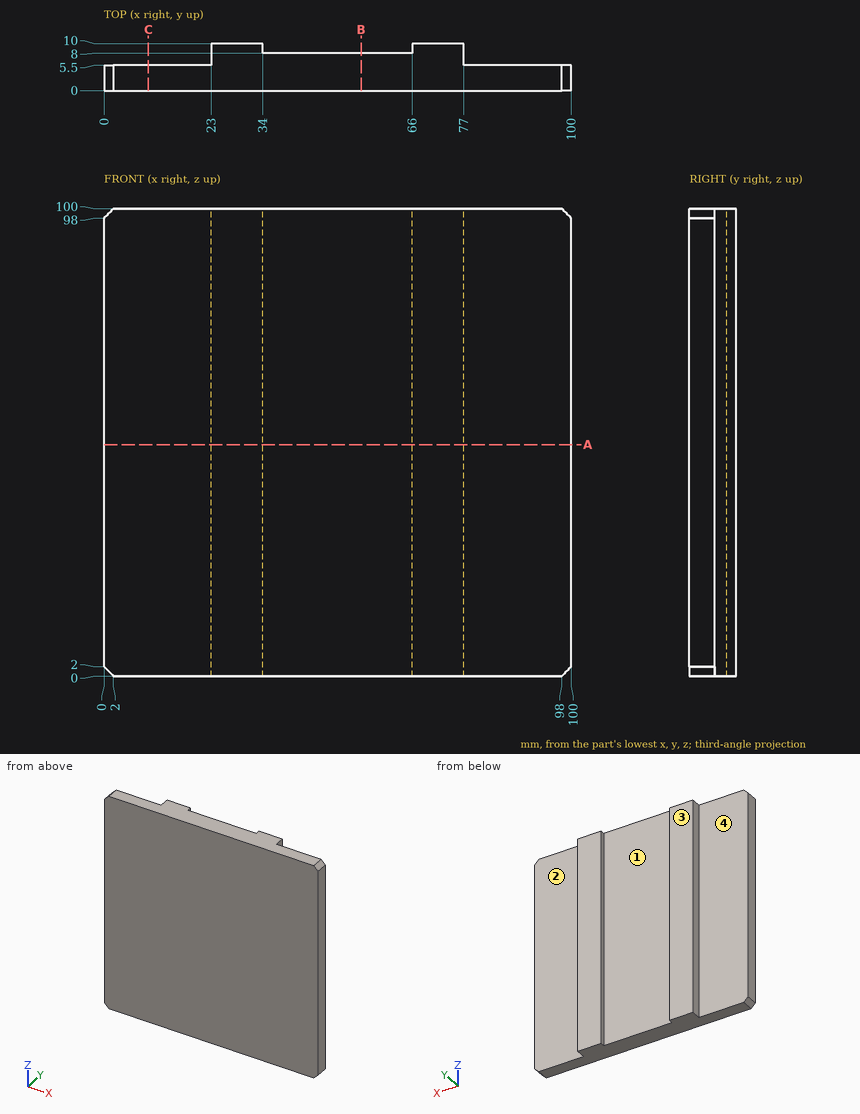
Verification items for this drawing (mm, ordinates from the low corner). A direction names the side the tool comes from. Give positions to 0.01 mm unless a question says otherwise; leave off trailing zeros. Loops run counter-clockwise (first coordinate to the right, second up) from the corner with the lowest first, then second, coordinate; pieces in that order, holes last.
(1) Depth check by flat-ended pin: pin 1 Ø2 at (y, z) = (7, 73.5) entering from +X; pin 2 Ø1 at (y, z) = (9.5, 64) entering from -X; pin 3 Ø16 at (x, z) = (49, 66) entering from +Y. Enter the tip coordinate at first touch or a pass-through.
From the geometry:
pin 1: stops at x = 77
pin 2: stops at x = 23
pin 3: stops at y = 8
(2) Set-up check for the marked faces 3 and 4: record each of +Z, -Z, +X, -X, +Y, -Y from which the full face is reachable in a straight line by a thin tool's end or side.
From the geometry:
face 3: +Z, -Z, +X, -X, +Y
face 4: +Z, -Z, -X, +Y
(3) Thickness scan on L1, parallel to X at y = 9, z = 48; L2, parallel to Y at x = 57, z = 83; L3, parallel to X at y = 6.5, z = 73. Record the ranges inside material, lowest first.
From the geometry:
L1: x = 23 to 34, 66 to 77
L2: y = 0 to 8
L3: x = 23 to 77
(4) Release check for a two-part mould opening along X. For the marked faces 1 and 2 record: released by +X, released by -X, zero draft, split by the parting line, or undercut.
From the geometry:
face 1: undercut
face 2: zero draft
(5) Section check C-C on x = 9.5. Record the cut outline in (y, z), then the cut area to 3 significant figures.
From the geometry:
outline: (0, 0) - (5.5, 0) - (5.5, 100) - (0, 100) - close
area: 550 mm2
(6) Section check A-A on z = 49.5. Record the cut outline in (x, y), then the cut area to 3 significant figures.
From the geometry:
outline: (0, 0) - (100, 0) - (100, 5.5) - (77, 5.5) - (77, 10) - (66, 10) - (66, 8) - (34, 8) - (34, 10) - (23, 10) - (23, 5.5) - (0, 5.5) - close
area: 729 mm2
(7) Section check B-B on x = 55. Record the cut outline in (y, z).
From the geometry:
outline: (0, 0) - (8, 0) - (8, 100) - (0, 100) - close
